from build123d import *

# Parameters (mm, degrees)
SKETCH1_R          = 12.5
EXTRUSION1_DEPTH   = 55
SKETCH2_R          = 13
EXTRUSION2_DEPTH   = 38.75
SKETCH3_R          = 7
EXTRUSION3_DEPTH   = 3
SKETCH4_R          = 2.5
EXTRUSION4_DEPTH   = 14.5
SKETCH5_R          = 1
EXTRUSION5_DEPTH   = 4
SKETCH6_R          = 4
EXTRUSION6_DEPTH   = 2.75
SKETCH7_R          = 1.5
EXTRUSION7_DEPTH   = 15
SKETCH8_W          = 0.4
SKETCH8_H          = 2.8
EXTRUSION8_DEPTH   = 8.7
CUT_EXTRUDE1_DEPTH = 10


with BuildPart() as part:
    # Sketch1 → Extrusion1 (new body)
    with BuildSketch(Plane.XY):
        Circle(SKETCH1_R)
    extrude(amount=EXTRUSION1_DEPTH)

    # Sketch2 → Extrusion2 (add)
    with BuildSketch(Plane.XY.offset(55)):
        Circle(SKETCH2_R)
    extrude(amount=EXTRUSION2_DEPTH)

    # Sketch3 → Extrusion3 (add)
    with BuildSketch(Plane.XY.offset(93.75)):
        with Locations(Location((0, 0, 0), (0, 0, 180))):
            Circle(SKETCH3_R)
    extrude(amount=EXTRUSION3_DEPTH)

    # Sketch4 → Extrusion4 (add)
    with BuildSketch(Plane.XY.offset(96.75)):
        Circle(SKETCH4_R)
    extrude(amount=EXTRUSION4_DEPTH)

    # Sketch5 → Extrusion5 (cut)
    with BuildSketch(Plane.XY.offset(93.75)):
        with Locations((0, 10)):
            Circle(SKETCH5_R)
        with Locations((10, 0)):
            Circle(SKETCH5_R)
        with Locations((0, -10)):
            Circle(SKETCH5_R)
        with Locations((-10, 0)):
            Circle(SKETCH5_R)
    extrude(amount=-EXTRUSION5_DEPTH, mode=Mode.SUBTRACT)

    # Sketch6 → Extrusion6 (add)
    with BuildSketch(Plane(origin=(0, 0, 0), x_dir=(-1, 0, 0), z_dir=(0, 0, -1))):
        Circle(SKETCH6_R)
    extrude(amount=EXTRUSION6_DEPTH)

    # Sketch7 → Extrusion7 (add)
    with BuildSketch(Plane(origin=(0, 0, 0), x_dir=(-1, 0, 0), z_dir=(0, 0, -1))):
        Circle(SKETCH7_R)
    extrude(amount=EXTRUSION7_DEPTH)

    # Sketch8 → Extrusion8 (add)
    with BuildSketch(Plane(origin=(0, 0, 0), x_dir=(-1, 0, 0), z_dir=(0, 0, -1))):
        with Locations((9.2, 0)):
            Rectangle(SKETCH8_W, SKETCH8_H)
        with Locations((-9.2, 0)):
            Rectangle(SKETCH8_W, SKETCH8_H)
    extrude(amount=EXTRUSION8_DEPTH)

    # Sketch9 → Cut-Extrude1 (cut)
    with BuildSketch(Plane.XY.offset(111.25)):
        Polygon((53.72529209, -1.5), (2, -1.5), (-2, -1.5), (-53.72529209, -1.5), (-53.72529209, -104.95058418), (53.72529209, -104.95058418), align=None)
    extrude(amount=-CUT_EXTRUDE1_DEPTH, mode=Mode.SUBTRACT)


solid = part.part
Geometry check sheet. Reference: the model listing, model coordinates, mm. A direction names the side the tool comes from. Round coordinates to 2 decimals unless told otherwise and drop trailing zeros. Loops run counter-clockwise (first coordinate to the right, second up) from the corner with the lowest first, then second, coordinate; pieces in that order, holes last.
Item 1: Access from +Z, -Z, +X, -X, +Y, -Y to the whole of each face (thin tool, end or side, straight path). Record for faces 5 (the flat face through (6, -6, 93.75)), 6 (the flat face through (9, 0, -4)), 7 (the flat face through (-2, 0, -2.75)).
Item 2: Cross-section at B-B on z = 44. Record the boundary of the cut face in (x, y).
Item 3: Mould release check, pull along Y, two halves, no side actions. Record for faces 1 (the cylindrical face through (-6.466, 2.681, 95.229)), 2 (the flat face through (10, 0, 89.75)), 3 (the flat face through (0, -1.5, 106)), 4 (the flat face through (9.4, 0, -4)): pulls with the +Y half, pulls with the -Y half, needs draft (parallel to the pull), parting line crosses it, or undercut.
Item 4: Gauge pin test, flat ends, axial feed: pin 1 (2 mm diameter, centred on x = 8, y = 7.5, fed in from -Z); pin 2 (12 mm diameter, centred on y = -8, z = 14.5, fed in from -X); pin 3 (3 mm diameter, centred on x = 10, y = 0, fed in from -Z); pin 4 (9 mm diameter, centred on x = -1.5, y = -1, fed in from -Z). Record the tip position at first contact, or that the pin passes through.
Item 5: Thickness scan on line 1 (Y direction, x = 0, z = 91.1); line 2 (Z direction, x = -2.75, y = -4.5); line 3 (Z direction, x = -8, y = 2.5). Record the ranges inside material, lowest first.
Item 6: Cross-section at A-A on x = -5.75. Record the boundary of the cut face in (y, z).
Answer sheet:
1. face 5: +Z
1. face 6: -Z, +Y, -Y
1. face 7: -Z
2. outline: circle Ø25 at (0, 0)
3. face 1: parting line crosses it
3. face 2: undercut
3. face 3: pulls with the -Y half
3. face 4: needs draft
4. pin 1: stops at z = 0
4. pin 2: stops at x = -12.34
4. pin 3: stops at z = -8.7
4. pin 4: stops at z = -15
5. line 1: y = -13 to -11, -9 to 9, 11 to 13
5. line 2: z = 0 to 96.75
5. line 3: z = 0 to 93.75
6. outline: (-11.66, 55) - (-11.1, 55) - (-11.1, 0) - (11.1, 0) - (11.1, 55) - (11.66, 55) - (11.66, 93.75) - (3.99, 93.75) - (3.99, 96.75) - (-3.99, 96.75) - (-3.99, 93.75) - (-11.66, 93.75) - close
